from build123d import *

# Parameters (mm, degrees)
CROQUIS3_W              = 750
CROQUIS3_H              = 500
SALIENTE_EXTRUIR1_DEPTH = 10
CROQUIS5_W              = 360
CROQUIS5_H              = 190
CORTAR_EXTRUIR2_DEPTH   = 2
CORTAR_EXTRUIR3_DEPTH   = 4
CROQUIS8_W              = 50
CROQUIS8_H              = 26.360948023
SALIENTE_EXTRUIR2_DEPTH = 15
CROQUIS9_W              = 160
CROQUIS9_H              = 52
SALIENTE_EXTRUIR3_DEPTH = 10


with BuildPart() as part:
    # Croquis3 → Saliente-Extruir1 (new body)
    with BuildSketch(Plane(origin=(0, 0, 0), x_dir=(1, 0, 0), z_dir=(0, 1, 0))):
        Rectangle(CROQUIS3_W, CROQUIS3_H)
    extrude(amount=-SALIENTE_EXTRUIR1_DEPTH)

    # Croquis5 → Cortar-Extruir2 (cut)
    with BuildSketch(Plane(origin=(0, 0, 0), x_dir=(1, 0, 0), z_dir=(0, 1, 0))):
        with Locations((-75, 105)):
            Rectangle(CROQUIS5_W, CROQUIS5_H)
        Polygon((-350, -60), (210, -60), (257.294818332, -60), (375, -142.41805549), (375, -250), (267.12592027, -250), (210, -210), (-350, -210), (-375, -227.505188455), (-375, -60), align=None)
    extrude(amount=-CORTAR_EXTRUIR2_DEPTH, mode=Mode.SUBTRACT)

    # Croquis7 → Cortar-Extruir3 (cut)
    with BuildSketch(Plane(origin=(0, -2, 0), x_dir=(1, 0, 0), z_dir=(0, 1, 0))):
        Polygon((318.412529557, -182.145430387), (334.795570442, -193.616959114), (323.324041715, -210), (306.94100083, -198.528471273), align=None)
    extrude(amount=-CORTAR_EXTRUIR3_DEPTH, mode=Mode.SUBTRACT)

    # Croquis8 → Saliente-Extruir2 (add)
    with BuildSketch(Plane.XZ.offset(10)):
        with Locations((-93.677785159, -94.090467316)):
            Rectangle(CROQUIS8_W, CROQUIS8_H)
    extrude(amount=SALIENTE_EXTRUIR2_DEPTH)

    # Croquis9 → Saliente-Extruir3 (add)
    with BuildSketch(Plane.XZ.offset(10)):
        with Locations((-148.677785159, -94.090467317)):
            Rectangle(CROQUIS9_W, CROQUIS9_H)
    extrude(amount=SALIENTE_EXTRUIR3_DEPTH)


solid = part.part
Geometry: final body of the model. Coordinates: model frame, mm. A direction names the side the tool comes from. Give positions to 0.01 mm unless a question says otherwise; leave off trailing zeros. Write each loop counter-clockwise with the first axis right and the second up, starting at its lowest first coordinate (ties: lowest second). Pieces come first, ordered by that corner, then holes.
(1) Cut plane B-B, the plane z = -155.5. Return loops of the section in (x, y), then the cut area to 3 significant figures.
(2) Mould query, pull axis Z, two halves, no side actions, for faces 6 (the flat face through (-362.325, -0.986, 218.63)), 7 (the flat face through (-58, 0, 230)). Classes: released by +Z, released by -Z, zero draft, split by the parting line, or undercut.
(3) Cut plane A-A, the plane x = 116.5. Return loops of the section in (y, z).
(4) Ray query, line 1 (Z direction, x = 92.5, y = -0.75); line 2 (Y direction, x = -293.5, z = 134); line 3 (Y direction, x = 278.5, z = -104). Return the intervals inside material, ascending.
(5) First-contact query: P1, Ø5.5, axis at x = -95, y = -22, coming from the +Z side; P2, Ø5.5, axis at x = -87.5, y = -22.5, coming from the -Z side; P3, Ø2, axis at x = -95, z = -67, coming from the -Y side. Flat tips, straight axial feed; report the tip coordinate or a pass-through.
(6) Cut plane C-C, the plane y = -16. Return loops of the section in (x, z), then the cut area to 3 significant figures.
(7) Access query for faces 1 (the flat face through (-5, 0, 31)), 2 (the flat face through (-78, -2, -106)), 3 (the flat face through (238.96, -0.99, 230.28)), 4 (the flat face through (-94, -25, -94)), 5 (the flat face through (-68.678, -16, -94)). Directions: +Z, -Z, +X, -X, +Y, -Y. A direction counts if a zero-diameter tool reaches every point of the face in a straight line with its end or side. Return the directions, or none.
Values follow:
1. outline: (-375, -10) - (375, -10) - (375, 0) - (105, 0) - (105, -2) - (-255, -2) - (-255, 0) - (-375, 0) - close
1. area: 6,780 mm2
2. face 6: undercut
2. face 7: zero draft
3. outline: (-10, -250) - (0, -250) - (0, 60) - (-2, 60) - (-2, 210) - (0, 210) - (0, 250) - (-10, 250) - close
4. line 1: z = -250 to -200, -10 to 60, 210 to 250
4. line 2: y = -10 to -2
4. line 3: y = -10 to 0
5. P1: stops at z = -68.09
5. P2: stops at z = -120.09
5. P3: stops at y = -10
6. outline: (-228.68, -120.09) - (-68.68, -120.09) - (-68.68, -68.09) - (-228.68, -68.09) - close
6. area: 8,320 mm2
7. face 1: +Z, -Z, +X, -X, +Y
7. face 2: +Y
7. face 3: +X, +Y
7. face 4: +Z, -Z, +X, -X, -Y
7. face 5: +Z, -Z, +X, -Y
